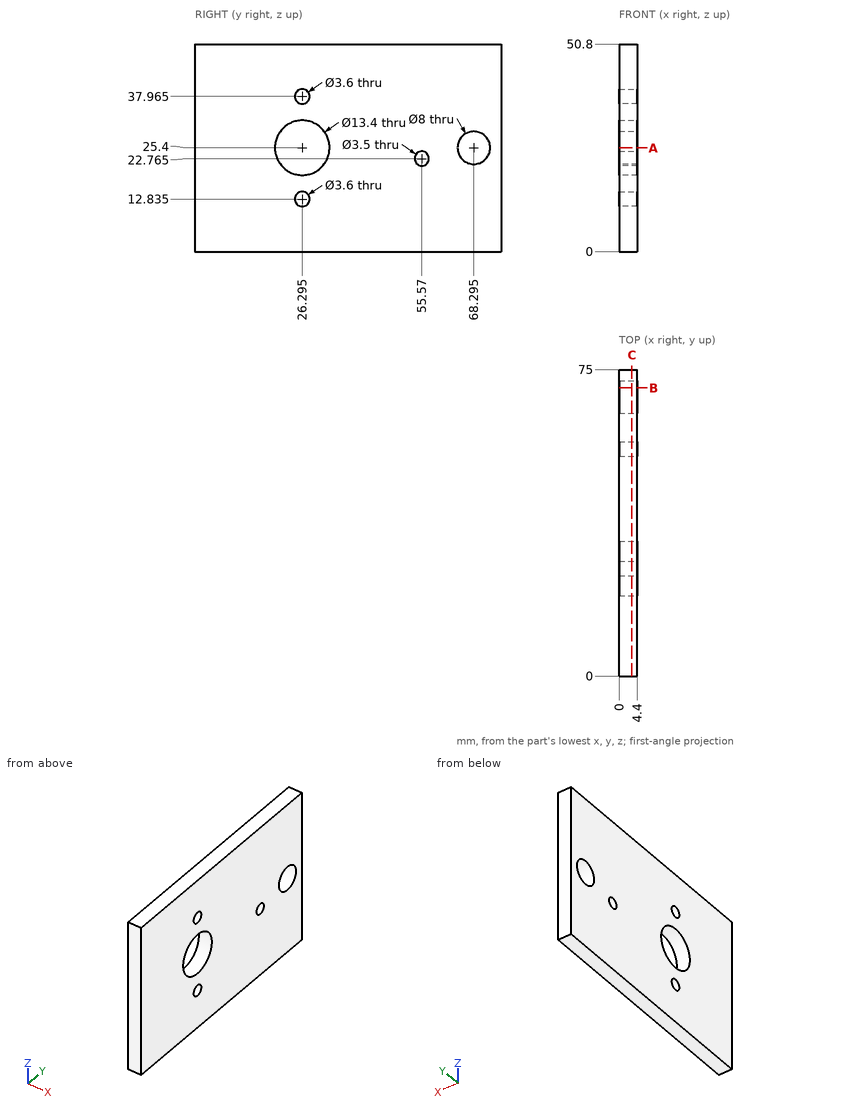
Source: three-view drawing plus pictorial views. Frame: mm from the lowest corner of the part. Give positions to 0.01 mm unless a question says otherwise; leave off trailing zeros. Order: outer loops, then holes, each group sorted by start corner. A loop starts at its lowest first (then second) coordinate and runs counter-clockwise, first axis right, second up. Notation, with made-up numbers: (35.25, 29) - (62.25, 29) arc R11 ccw to (62.25, 42) - close; hole circle Ø8 at (-30, 33). An arc over 180 degrees is marked (long way). Answer as a JSON object with one key per item and string values. Group by question number.
Q1. Cut plane B-B, the plane y = 70.5. Output: boundary loops of the cut face in (x, z).
Q2. Cut plane A-A, the plane z = 25.4. Output: boundary loops of the cut face in (x, y) (1 decimal), then the cut area to 3 significant figures.
Q3. Cut plane C-C, the plane x = 3.1. Count the separate pieces of the cut face and the enclosed holes in it, then the cut area to 3 significant figures.
Q4. Line query: probe 1 along Y at (x, z) = (3.05, 25.4) (1 decimal); probe 2 along Y at (x, z) = (3.2, 28) (1 decimal); probe 3 along Z at (x, y) = (1.55, 66) (1 decimal). Output: solid intervals per line, ascending.
Q5. First-contact query: pin 1 Ø10.5 at (y, z) = (26.29, 25.4) entering from +X. Flat tip, straight axial feed; report the tip coordinate or a pass-through.
Results:
{
 "1": {"outline": "(0, 0) - (4.4, 0) - (4.4, 22.06) - (0, 22.06) - close; (0, 28.74) - (4.4, 28.74) - (4.4, 50.8) - (0, 50.8) - close"},
 "2": {"outline": "(0, 0) - (4.4, 0) - (4.4, 19.6) - (0, 19.6) - close; (0, 33) - (4.4, 33) - (4.4, 64.3) - (0, 64.3) - close; (0, 72.3) - (4.4, 72.3) - (4.4, 75) - (0, 75) - close", "area": "236 mm^2"},
 "3": {"separate pieces": "1", "enclosed holes": "5", "area": "3,590 mm^2"},
 "4": {"probe 1": "0 to 19.6, 33 to 64.3, 72.3 to 75", "probe 2": "0 to 20.1, 32.5 to 65.3, 71.3 to 75", "probe 3": "0 to 22.1, 28.7 to 50.8"},
 "5": {"pin 1": "through"}
}
